Model file for the job. Use its own axes, mm. Coordinates: 2 decimals unless noted, no trailing zeros. Loops run counter-clockwise (first coordinate to the right, second up) from the corner with the lowest first, then second, coordinate; pieces in that order, holes last.
from build123d import *

# Parameters (mm, degrees)
SKETCH1_W                       = 152.4
SKETCH1_H                       = 254
BOSS_EXTRUDE1_DEPTH             = 1.27
SKETCH2_R                       = 14.2875
UPPER_INTAKE_BEARING_HOLE_DEPTH = 2.54
SKETCH3_R                       = 14.2875
LOWER_INTAKE_BEARING_HOLE_DEPTH = 2.54


with BuildPart() as part:
    # Sketch1 → Boss-Extrude1 (new, symmetric)
    with BuildSketch(Plane(origin=(0, 0, 0), x_dir=(0, 0, -1), z_dir=(1, 0, 0))):
        Rectangle(SKETCH1_W, SKETCH1_H)
    extrude(amount=BOSS_EXTRUDE1_DEPTH, both=True)

    # Sketch2 → upper intake bearing hole (cut)
    with BuildSketch(Plane(origin=(1.27, 0, 0), x_dir=(0, 0, -1), z_dir=(1, 0, 0))):
        with Locations((-25.4, -25.4)):
            Circle(SKETCH2_R)
    extrude(amount=-UPPER_INTAKE_BEARING_HOLE_DEPTH, mode=Mode.SUBTRACT)

    # Sketch3 → lower intake bearing hole (cut)
    with BuildSketch(Plane(origin=(1.27, 0, 0), x_dir=(0, 0, -1), z_dir=(1, 0, 0))):
        with Locations((50.8, -104.775)):
            Circle(SKETCH3_R)
    extrude(amount=-LOWER_INTAKE_BEARING_HOLE_DEPTH, mode=Mode.SUBTRACT)


solid = part.part
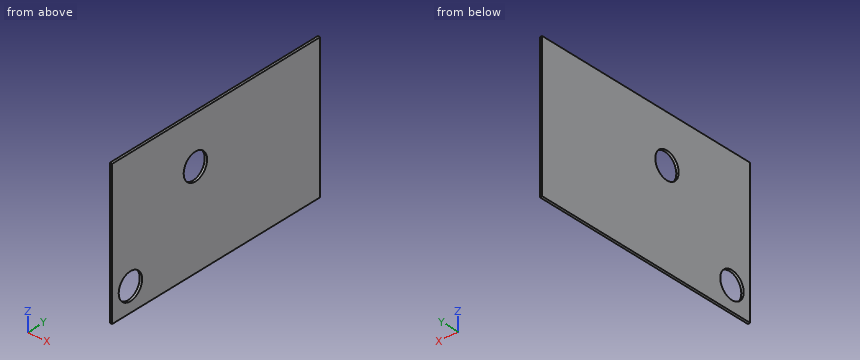
Q1. Slice it at C-C (x = 0.6). List the corners of the cut face in (y, z) (1 decimal).
Answers:
outline: (-127, -76.2) - (127, -76.2) - (127, 76.2) - (-127, 76.2) - close; hole circle Ø28.6 at (-104.8, -50.8); hole circle Ø28.6 at (-25.4, 25.4)
Q2. Drill centre lines: line 1 (Y direction, x = -0.1, z = -50.8); line 2 (Y direction, x = 0.8, z = 25.4); line 3 (Z direction, x = 0.2, y = -22). Where is each one in solid material? Low to high.
Answers:
line 1: y = -127 to -119.06, -90.49 to 127
line 2: y = -127 to -39.69, -11.11 to 127
line 3: z = -76.2 to 11.52, 39.28 to 76.2
Q3. Slice it at A-A (z = -50.8). List the corners of the cut face in (x, y).
Answers:
outline: (-1.27, -127) - (1.27, -127) - (1.27, -119.06) - (-1.27, -119.06) - close; (-1.27, -90.49) - (1.27, -90.49) - (1.27, 127) - (-1.27, 127) - close
Q4. Slice it at B-B (y = -25.4). List the corners of the cut face in (x, z), and give its area (3 significant figures).
Answers:
outline: (-1.27, -76.2) - (1.27, -76.2) - (1.27, 11.11) - (-1.27, 11.11) - close; (-1.27, 39.69) - (1.27, 39.69) - (1.27, 76.2) - (-1.27, 76.2) - close
area: 315 mm2
